```python
from build123d import *

# Parameters (mm, degrees)
CROQUIS1_R              = 2
SALIENTE_EXTRUIR2_DEPTH = 100
MOVE_FACE_1_BY          = 135


with BuildPart() as part:
    # Croquis1 → Saliente-Extruir2 (new body)
    with BuildSketch(Plane.XY):
        with BuildLine():
            Line((-4.825, 10), (-3.125, 8.3))
            Line((-3.125, 8.3), (-5.5, 8.3))
            Line((-5.5, 8.3), (-5.5, 6.560660172))
            Line((-5.5, 6.560660172), (-2.939339828, 4))
            Line((-2.939339828, 4), (2.939339828, 4))
            Line((2.939339828, 4), (5.5, 6.560660172))
            Line((5.5, 6.560660172), (5.5, 8.3))
            Line((5.5, 8.3), (3.125, 8.3))
            Line((3.125, 8.3), (4.825, 10))
            Line((4.825, 10), (9.5, 10))
            ThreePointArc((9.5, 10), (9.853553391, 9.853553391), (10, 9.5))
            Line((10, 9.5), (10, 4.825))
            Line((10, 4.825), (8.3, 3.125))
            Line((8.3, 3.125), (8.3, 5.5))
            Line((8.3, 5.5), (6.560660172, 5.5))
            Line((6.560660172, 5.5), (4, 2.939339828))
            Line((4, 2.939339828), (4, -2.939339828))
            Line((4, -2.939339828), (6.560660172, -5.5))
            Line((6.560660172, -5.5), (8.3, -5.5))
            Line((8.3, -5.5), (8.3, -3.125))
            Line((8.3, -3.125), (10, -4.825))
            Line((10, -4.825), (10, -9.5))
            ThreePointArc((10, -9.5), (9.853553391, -9.853553391), (9.5, -10))
            Line((9.5, -10), (4.825, -10))
            Line((4.825, -10), (3.125, -8.3))
            Line((3.125, -8.3), (5.5, -8.3))
            Line((5.5, -8.3), (5.5, -6.560660172))
            Line((5.5, -6.560660172), (2.939339828, -4))
            Line((2.939339828, -4), (-2.939339828, -4))
            Line((-2.939339828, -4), (-5.5, -6.560660172))
            Line((-5.5, -6.560660172), (-5.5, -8.3))
            Line((-5.5, -8.3), (-3.125, -8.3))
            Line((-3.125, -8.3), (-4.825, -10))
            Line((-4.825, -10), (-9.5, -10))
            ThreePointArc((-9.5, -10), (-9.853553391, -9.853553391), (-10, -9.5))
            Line((-10, -9.5), (-10, -4.825))
            Line((-10, -4.825), (-8.3, -3.125))
            Line((-8.3, -3.125), (-8.3, -5.5))
            Line((-8.3, -5.5), (-6.560660172, -5.5))
            Line((-6.560660172, -5.5), (-4, -2.939339828))
            Line((-4, -2.939339828), (-4, 2.939339828))
            Line((-4, 2.939339828), (-6.560660172, 5.5))
            Line((-6.560660172, 5.5), (-8.3, 5.5))
            Line((-8.3, 5.5), (-8.3, 3.125))
            Line((-8.3, 3.125), (-10, 4.825))
            Line((-10, 4.825), (-10, 9.5))
            ThreePointArc((-10, 9.5), (-9.853553391, 9.853553391), (-9.5, 10))
            Line((-9.5, 10), (-4.825, 10))
        make_face()
        Circle(CROQUIS1_R, mode=Mode.SUBTRACT)
    extrude(amount=SALIENTE_EXTRUIR2_DEPTH)

    # Move Face 1: a face moved outward by 135.0
    extrude(part.faces().sort_by_distance((5, -5, 0))[0], amount=MOVE_FACE_1_BY, dir=(0, 0, -1))


solid = part.part
```
Geometry check sheet. Reference: the model listing, model coordinates, mm. A direction names the side the tool comes from. Round coordinates to 2 decimals unless told otherwise and drop trailing zeros. Order: outer loops, then holes, each group sorted by start corner. A loop starts at its lowest first (then second) coordinate and runs counter-clockwise, first axis right, second up. Notation, with made-up numbers: M 24.25,53 L 35.25,53 A24 ccw 35.25,78 Z; hole C 59,85.5 d11. An arc over 180 degrees is marked long. Answer as CSV lines item,"result".
1) Tool access check on faces 4 (the face through (-4, 0, -16)), 5 (the face through (0, -2, -19)), 6 (the face through (0, 4, -16)), 7 (the face through (4, 0, -16)). Record the directions out of +Z, -Z, +X, -X, +Y, -Y that give a thin tool (end or side, any length) a straight path to the whole face; none if there is none.
Entries:
face 4,"+Z, -Z, -X"
face 5,"+Z, -Z"
face 6,"+Z, -Z, +Y"
face 7,"+Z, -Z, +X"
2) Gauge pin test, flat ends, axial feed: pin 1 Ø3 at (x, z) = (-0.5, -72.5) entering from +Y; pin 2 Ø6.5 at (y, z) = (-0.5, 27) entering from -X (3 decimals); pin 3 Ø0.7 at (y, z) = (-4, -10) entering from +X (3 decimals); pin 4 Ø1.5 at (x, y) = (3, 7.5) entering from +Z. Record the tip position at first contact, or that the pin passes through.
Entries:
pin 1,"y = 4"
pin 2,"x = -8.925"
pin 3,"x = 9.525"
pin 4,"through"
3) Sectioned sample at A-A on x = 0. Record the cut outline in (y, z), and give its area (3 significant figures).
Entries:
outline,"M -4,-135 L -2,-135 L -2,100 L -4,100 Z; M 2,-135 L 4,-135 L 4,100 L 2,100 Z"
area,"940 mm2"
4) Thickness scan on probe 1 along Y at (x, z) = (0, -58); probe 2 along X at (y, z) = (7, -44); probe 3 along Y at (x, z) = (-4.75, -91.5) (3 decimals). Record the ranges inside material, lowest first. Write a range as [from, to].
Entries:
probe 1,"[-4, -2], [2, 4]"
probe 2,"[-10, -5.5], [5.5, 10]"
probe 3,"[-9.925, -8.3], [-5.811, -3.689], [3.689, 5.811], [8.3, 9.925]"
5) Mould release check, pull along X, two halves, no side actions. Record for faces 1 (the face through (0, -4, -16)), 2 (the face through (10, 7, -16)), 3 (the face through (-7, -10, -16)): +X half, -X half, draft (parallel to the pull), parting line (faces both ways), or undercut.
Entries:
face 1,"undercut"
face 2,"+X half"
face 3,"draft"
